Source: CAD feature listing. Evaluate the final solid. Frame: model axes, mm. Face numbers are marked on the shaded views. A direction names the side the tool comes from. Coordinates: 2 decimals unless noted, no trailing zeros. Order: outer loops, then holes, each group sorted by start corner. A loop starts at its lowest first (then second) coordinate and runs counter-clockwise, first axis right, second up. Notation, with made-up numbers: (48.25, 85) - (71.25, 85) arc R33 ccw to (71.25, 114) - close; hole circle Ø8 at (66.25, 6). An arc over 180 degrees is marked (long way). One line per question, with ' | ' between items. Start each with the question number.
(1) Section C-C (x = 55). Return the cut outline in (y, z), then the cut area to 3 significant figures.
(2) Contact query for flat-ended pins moving along their axis: P1, Ø8, axis at y = -1, z = 194.5, coming from the +X side; P2, Ø5, axis at y = 7, z = 212, coming from the -X side; P3, Ø0.5, axis at x = -30, y = 57.5, coming from the +Z side. Output: stop coordinate, or through.
(3) Access query for the marked faces 5, 6, 7 and 8. Directions: +Z, -Z, +X, -X, +Y, -Y. A direction counts if a zero-diameter tool reaches every point of the face in a straight line with its end or side. Return the directions, or none.
(4) Section A-A (x = -10.5). Return the cut outline in (y, z), then the cut area to 3 significant figures.
(5) Draft query along Y for the marked faces 1, 2, 3 and 4. Return one class per face: +Y half, -Y half, draft (parallel to the pull), parting line (faces both ways), or undercut.
(6) Section B-B (y = 40). Return the cut outline in (x, z).
(7) Section D-D (z = 210.75). Count the separate pieces of the cut face and the enclosed holes in it, then the cut area to 3 significant figures.
(8) Line query: line 1 along X through (y, z) = (-5, 216.75); line 2 along Y through (x, z) = (-14.5, 191.25); line 3 along Y through (x, z) = (26, 216.25). Output: solid intervals per line, ascending.
from build123d import *

# Parameters (mm, degrees)
AUFSATZ_LINEAR_AUSTRAGEN1_DEPTH = 30
SKIZZE4_W                       = 19.059709953
SKIZZE4_H                       = 53.604548155
SCHNITT_LINEAR_AUSTRAGEN1_DEPTH = 1
SKIZZE5_W                       = 13.535379209
SKIZZE5_H                       = 6.598473738
SKIZZE5_W_2                     = 19.010784176
SKIZZE5_H_2                     = 9.525951679
SKIZZE5_W_3                     = 8.081851555
SKIZZE5_H_3                     = 9.33
SCHNITT_LINEAR_AUSTRAGEN2_DEPTH = 1
SKIZZE6_W                       = 11.254395851
SKIZZE6_H                       = 21.878706828
SCHNITT_LINEAR_AUSTRAGEN3_DEPTH = 1
SKIZZE8_W                       = 70.5
SKIZZE8_H                       = 18.817969375
SCHNITT_LINEAR_AUSTRAGEN4_DEPTH = 1
SCHNITT_LINEAR_AUSTRAGEN5_DEPTH = 18


with BuildPart() as part:
    # Skizze2 → Aufsatz-Linear austragen1 (new body)
    with BuildSketch(Plane(origin=(0, 0, 188.684819625), x_dir=(-1, 0, 0), z_dir=(0, 0, -1))):
        with BuildLine():
            Line((114.255256192, 57.804225359), (-71.202450647, 57.804225359))
            ThreePointArc((-71.202450647, 57.804225359), (-75.616222333, 55.975981265), (-77.444466427, 51.562209578))
            Line((-77.444466427, 51.562209578), (-77.444466427, 27.181394091))
            ThreePointArc((-77.444466427, 27.181394091), (-75.616222333, 22.767622404), (-71.202450647, 20.93937831))
            Line((-71.202450647, 20.93937831), (-23.9356809, 20.93937831))
            ThreePointArc((-23.9356809, 20.93937831), (-22.875020729, 20.500038482), (-22.4356809, 19.43937831))
            Line((-22.4356809, 19.43937831), (-22.4356809, -31.865246208))
            ThreePointArc((-22.4356809, -31.865246208), (-21.117661416, -35.047226723), (-17.9356809, -36.365246208))
            Line((-17.9356809, -36.365246208), (60.988486446, -36.365246208))
            ThreePointArc((60.988486446, -36.365246208), (64.170466961, -35.047226723), (65.488486446, -31.865246208))
            Line((65.488486446, -31.865246208), (65.488486446, 19.43937831))
            ThreePointArc((65.488486446, 19.43937831), (65.927826274, 20.500038482), (66.988486446, 20.93937831))
            Line((66.988486446, 20.93937831), (114.255256192, 20.93937831))
            ThreePointArc((114.255256192, 20.93937831), (118.669027879, 22.767622404), (120.497271973, 27.181394091))
            Line((120.497271973, 27.181394091), (120.497271973, 51.562209578))
            ThreePointArc((120.497271973, 51.562209578), (118.669027879, 55.975981265), (114.255256192, 57.804225359))
        make_face()
        with BuildLine():
            Line((114.255256192, 56.804225359), (-71.202450647, 56.804225359))
            ThreePointArc((-71.202450647, 56.804225359), (-74.909115552, 55.268874484), (-76.444466427, 51.562209578))
            Line((-76.444466427, 51.562209578), (-76.444466427, 27.181394091))
            ThreePointArc((-76.444466427, 27.181394091), (-74.909115552, 23.474729185), (-71.202450647, 21.93937831))
            Line((-71.202450647, 21.93937831), (-23.9356809, 21.93937831))
            ThreePointArc((-23.9356809, 21.93937831), (-22.167913947, 21.207145263), (-21.4356809, 19.43937831))
            Line((-21.4356809, 19.43937831), (-21.4356809, -31.865246208))
            ThreePointArc((-21.4356809, -31.865246208), (-20.410554634, -34.340119942), (-17.9356809, -35.365246208))
            Line((-17.9356809, -35.365246208), (60.988486446, -35.365246208))
            ThreePointArc((60.988486446, -35.365246208), (63.46336018, -34.340119942), (64.488486446, -31.865246208))
            Line((64.488486446, -31.865246208), (64.488486446, 19.43937831))
            ThreePointArc((64.488486446, 19.43937831), (65.220719493, 21.207145263), (66.988486446, 21.93937831))
            Line((66.988486446, 21.93937831), (114.255256192, 21.93937831))
            ThreePointArc((114.255256192, 21.93937831), (117.961921098, 23.474729185), (119.497271973, 27.181394091))
            Line((119.497271973, 27.181394091), (119.497271973, 51.562209578))
            ThreePointArc((119.497271973, 51.562209578), (117.961921098, 55.268874484), (114.255256192, 56.804225359))
        make_face(mode=Mode.SUBTRACT)
    extrude(amount=-AUFSATZ_LINEAR_AUSTRAGEN1_DEPTH)

    # Skizze4 → Schnitt-Linear austragen1 (cut)
    with BuildSketch(Plane(origin=(22.4356809, 0, 0), x_dir=(0, 0, -1), z_dir=(1, 0, 0))):
        with Locations((-204.849070455, -6.494967379)):
            Rectangle(SKIZZE4_W, SKIZZE4_H)
    extrude(amount=-SCHNITT_LINEAR_AUSTRAGEN1_DEPTH, mode=Mode.SUBTRACT)

    # Skizze5 → Schnitt-Linear austragen2 (cut)
    with BuildSketch(Plane.XZ.offset(36.365246208)):
        with Locations((-53.389754229, 198.342500668)):
            Rectangle(SKIZZE5_W, SKIZZE5_H)
        with Locations((-32.103878534, 199.806239639)):
            Rectangle(SKIZZE5_W_2, SKIZZE5_H_2)
        with Locations((-10.407185504, 199.904215478)):
            Rectangle(SKIZZE5_W_3, SKIZZE5_H_3)
    extrude(amount=-SCHNITT_LINEAR_AUSTRAGEN2_DEPTH, mode=Mode.SUBTRACT)

    # Skizze6 → Schnitt-Linear austragen3 (cut)
    with BuildSketch(Plane.ZY.offset(65.488486446)):
        with Locations((199.312017551, -5.205318356)):
            Rectangle(SKIZZE6_W, SKIZZE6_H)
    extrude(amount=-SCHNITT_LINEAR_AUSTRAGEN3_DEPTH, mode=Mode.SUBTRACT)

    # Skizze8 → Schnitt-Linear austragen4 (cut)
    with BuildSketch(Plane(origin=(0, 57.804225359, 0), x_dir=(1, 0, 0), z_dir=(0, 1, 0))):
        with Locations((-21.082442705, -210.135508824)):
            Rectangle(SKIZZE8_W, SKIZZE8_H)
    extrude(amount=-SCHNITT_LINEAR_AUSTRAGEN4_DEPTH, mode=Mode.SUBTRACT)

    # Skizze9 → Schnitt-Linear austragen5 (cut)
    with BuildSketch(Plane.XY.offset(218.684819625)):
        with BuildLine():
            Line((77.444466427, 51.562209578), (77.444466427, 27.181394091))
            ThreePointArc((77.444466427, 27.181394091), (75.616222333, 22.767622404), (71.202450647, 20.93937831))
            Line((71.202450647, 20.93937831), (42.046255802, 20.93937831))
            Line((42.046255802, 20.93937831), (42.046255802, 57.804225359))
            Line((42.046255802, 57.804225359), (71.202450647, 57.804225359))
            ThreePointArc((71.202450647, 57.804225359), (75.616222333, 55.975981265), (77.444466427, 51.562209578))
        make_face()
        with BuildLine():
            Line((-85.099061347, 57.804225359), (-85.099061347, 20.93937831))
            Line((-85.099061347, 20.93937831), (-114.255256192, 20.93937831))
            ThreePointArc((-114.255256192, 20.93937831), (-118.669027879, 22.767622404), (-120.497271973, 27.181394091))
            Line((-120.497271973, 27.181394091), (-120.497271973, 51.562209578))
            ThreePointArc((-120.497271973, 51.562209578), (-118.669027879, 55.975981265), (-114.255256192, 57.804225359))
            Line((-114.255256192, 57.804225359), (-85.099061347, 57.804225359))
        make_face()
    extrude(amount=-SCHNITT_LINEAR_AUSTRAGEN5_DEPTH, mode=Mode.SUBTRACT)


solid = part.part
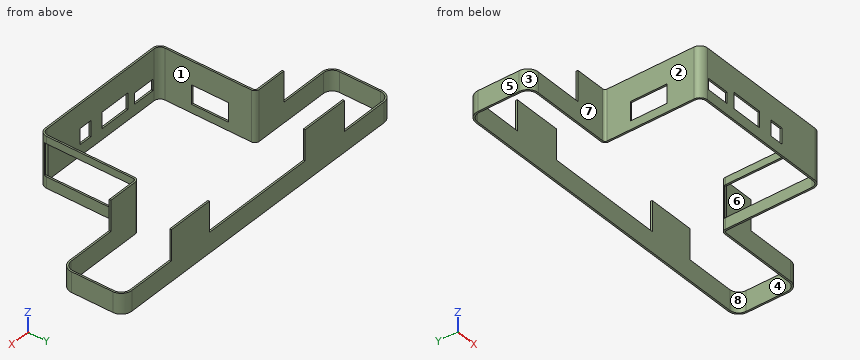
Response values:
1) outline: (20.94, 188.68) - (21.94, 188.68) - (21.94, 200.68) - (20.94, 200.68) - close; (56.8, 188.68) - (57.8, 188.68) - (57.8, 200.68) - (56.8, 200.68) - close | area: 24.0 mm²
2) P1: stops at x = 22.44 | P2: stops at x = -65.49 | P3: stops at z = 200.73
3) face 5: +Z, -Z, -X, +Y, -Y | face 6: +Z, -Z, +X, -Y | face 7: +Z, -Z, -X, -Y | face 8: +Z, -Z
4) outline: (-36.37, 188.68) - (-35.37, 188.68) - (-35.37, 195.24) - (-36.37, 195.24) - close; (-36.37, 204.57) - (-35.37, 204.57) - (-35.37, 218.68) - (-36.37, 218.68) - close; (56.8, 188.68) - (57.8, 188.68) - (57.8, 200.73) - (56.8, 200.73) - close | area: 32.7 mm²
5) face 1: undercut | face 2: draft | face 3: -Y half | face 4: undercut
6) outline: (-120.5, 188.68) - (-119.5, 188.68) - (-119.5, 200.68) - (-120.5, 200.68) - close; (76.44, 188.68) - (77.44, 188.68) - (77.44, 200.68) - (76.44, 200.68) - close
7) separate pieces: 4 | enclosed holes: 0 | area: 240 mm²
8) line 1: x = -65.49 to -64.49, 21.44 to 22.44 | line 2: y = -36.37 to -35.37, 56.8 to 57.8 | line 3: y = 20.94 to 21.94, 56.8 to 57.8
